Source: CAD feature listing. Evaluate the final solid. Frame: model axes, mm. A direction names the side the tool comes from. Give positions to 0.01 mm unless a question says otherwise; leave off trailing zeros. Order: outer loops, then holes, each group sorted by start corner. A loop starts at its lowest first (then second) coordinate and runs counter-clockwise, first axis right, second up.
Autodesk Inventor part; units mm, degrees
ref_plane "YZ Plane" through (0, 0, 0) normal (1, 0, 0) x (0, 1, 0)
ref_plane "XZ Plane" through (0, 0, 0) normal (0, 1, 0) x (-1, 0, 0)
ref_plane "XY Plane" through (0, 0, 0) normal (0, 0, 1) x (1, 0, 0)
sketch "Sketch1" plane through (0, 0, 0) normal (0, 1, 0) x (-1, 0, 0)
  circle A0 centre (0, 0) radius 30
  dimension "d0" = 60
extrude "Extrusion1" add sketch "Sketch1" along normal blind 6
fillet "Fillet1" radius 6 1 edges at (30, 6, 0)
sketch "Sketch2" plane through (0, 0, 0) normal (0, -1, 0) x (1, 0, 0)
  line L0 (-7, -25) -> (7, -25)
  line L1 (7, -25) -> (7, -18)
  line L2 (7, -18) -> (-7, -18)
  line L3 (-7, -18) -> (-7, -25)
  line L4 (-7, -25) -> (7, -18) construction
  line L5 (7, -25) -> (-7, -18) construction
  arc A0 (-4.5, -25) -> (-9.5, -25) centre (-7, -25) ccw
  arc A1 (9.5, -25) -> (4.5, -25) centre (7, -25) ccw
  line L6 (-9.5, -25) -> (9.5, -25)
  point P0 (0, 0)
  point P1 (0, -21.5)
  dimension "d4" = 14
  dimension "d5" = 7
  dimension "d6" = 18
  dimension "d7" = 5
  dimension "d8" = 5
revolve "Revolution1" cut sketch "Sketch2" angle 360 about axis through (-7, 0, -25) along (1, 0, 0)
pattern_circular "Circular Pattern1" count 4 over 360 about axis through (0, -10, 0) along (0, 1, 0) of "Revolution1"
properties part number "omni_wheel_cover_template"
1) Reachability of faces 4 (the face through (24, 3, -7)), 5 (the face through (7, 3, -24)), 6 (the face through (-18.88, 3.4, 0.1)), 7 (the face through (7, 3, 24)) from +Z, -Z, +X, -X, +Y, -Y: full face, straight path, thin tool, end or side. Return the list, or none.
Checks:
face 4: +X, -Y
face 5: -Z, -Y
face 6: -X, -Y
face 7: +Z, -Y
2) Ray query, L1, parallel to X at y = 0.5, z = -21; L2, parallel to X at y = 1, z = -8; L3, parallel to Z at x = 25, y = 3.5. Return the intervals inside material, ascending.
Checks:
L1: x = -21.4 to -7, 7 to 21.4
L2: x = -28.83 to -27.06, -22.94 to 22.94, 27.06 to 28.83
L3: z = -14.45 to -7, 7 to 14.45
3) Section query D-D on y = 4.75. Output: boundary loops of the cut face in (x, z), and give its area (3 significant figures).
Checks:
outline: (-26.77, -7) arc R27.67 ccw to (-7, -26.77) - (-7, -19.86) - (7, -19.86) - (7, -26.77) arc R27.67 ccw to (26.77, -7) - (19.86, -7) - (19.86, 7) - (26.77, 7) arc R27.67 ccw to (7, 26.77) - (7, 19.86) - (-7, 19.86) - (-7, 26.77) arc R27.67 ccw to (-26.77, 7) - (-19.86, 7) - (-19.86, -7) - close
area: 1,980 mm2
4) Section query B-B on x = -3.5. Output: boundary loops of the cut face in (y, z), and give its area (3 significant figures).
Checks:
outline: (0, -18) arc R7 cw to (6, -21.39) - (6, 21.39) arc R7 cw to (0, 18) - close
area: 228 mm2
5) Pull-direction query (Z, two-part tool) for faces 1 (the face through (-24, 3, 7)), 2 (the face through (0.1, 3.4, 18.88)), 3 (the face through (0, 0, 0)); classes: +Z half, -Z half, draft (parallel to the pull), parting line (faces both ways), or undercut.
Checks:
face 1: undercut
face 2: +Z half
face 3: draft
6) First-contact query: pin 1 Ø1.8 at (x, y) = (22.5, 2.5) entering from -Z; pin 2 Ø2 at (x, y) = (20.5, 1.5) entering from +Z; pin 3 Ø1 at (x, y) = (4.5, 2) entering from +Z. Flat tips, straight axial feed; report the tip coordinate or a pass-through.
Checks:
pin 1: stops at z = -20.17
pin 2: stops at z = 22.6
pin 3: stops at z = 18.46
7) Section query C-C on z = -1. Output: boundary loops of the cut face in (x, y), and give its area (3 significant figures).
Checks:
outline: (-21.39, 6) arc R7 cw to (-18, 0) - (18, 0) arc R7 cw to (21.39, 6) - close
area: 228 mm2
